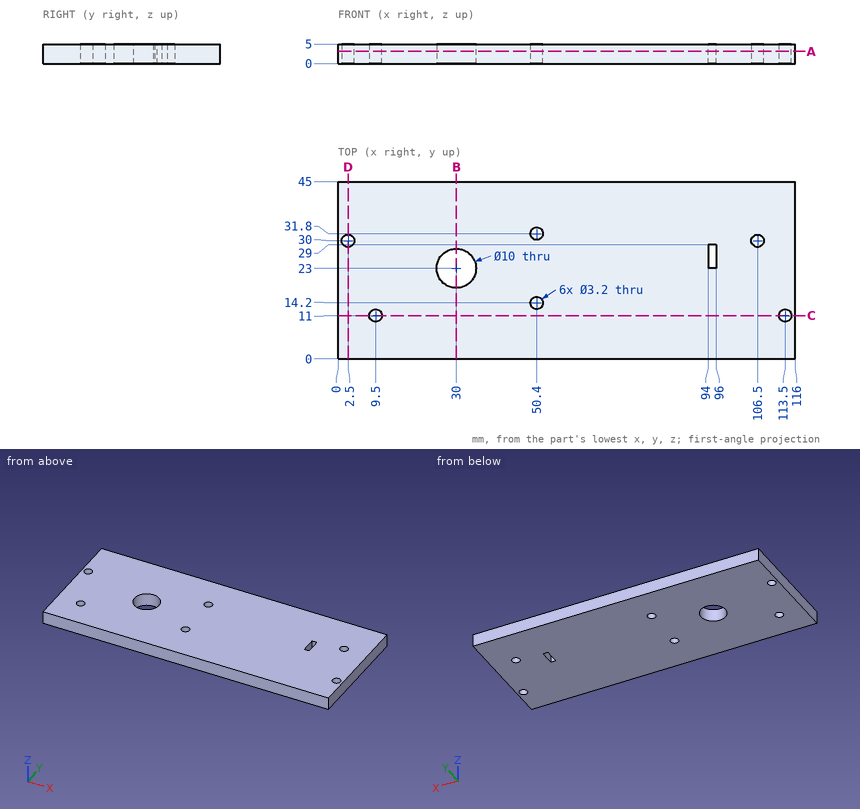
For this review, use the dimensioned drawing (mm, ordinates from the lowest corner) and the shaded views. Give positions to 0.01 mm unless a question says otherwise; leave off trailing zeros. Loops run counter-clockwise (first coordinate to the right, second up) from the corner with the lowest first, then second, coordinate; pieces in that order, holes last. Notation, with made-up numbers: (88.25, 46) -> (98.25, 46) arc R24 ccw to (98.25, 83) -> close; hole circle Ø10 at (7, -21). An arc over 180 degrees is marked (long way). One line per question, with ' | ' between items. Start each with the question number.
(1) We need section B-B (x = 30). State the section outline as (y, z) points, and give its area (3 significant figures).
(2) We need section D-D (x = 2.5). State the section outline as (y, z) points, and give its area (3 significant figures).
(3) We need section A-A (z = 3.15). State how many separate pieces and enclosed holes the cut face has, and give its area (3 significant figures).
(4) We need section C-C (y = 11). State the section outline as (x, z) points.
(5) For line 1 (X direction, y = 30, z = 2.95); line 2 (Y direction, x = 50.4, z = 2.7); line 3 (X direction, y = 11, z = 1.1), list the stretches that pass through material, from the lowest coordinate up.
The answers:
1) outline: (0, 0) -> (18, 0) -> (18, 5) -> (0, 5) -> close; (28, 0) -> (45, 0) -> (45, 5) -> (28, 5) -> close | area: 175 mm^2
2) outline: (0, 0) -> (28.4, 0) -> (28.4, 5) -> (0, 5) -> close; (31.6, 0) -> (45, 0) -> (45, 5) -> (31.6, 5) -> close | area: 209 mm^2
3) separate pieces: 1 | enclosed holes: 8 | area: 5,080 mm^2
4) outline: (0, 0) -> (7.9, 0) -> (7.9, 5) -> (0, 5) -> close; (11.1, 0) -> (111.9, 0) -> (111.9, 5) -> (11.1, 5) -> close; (115.1, 0) -> (116, 0) -> (116, 5) -> (115.1, 5) -> close
5) line 1: x = 0 to 0.9, 4.1 to 104.9, 108.1 to 116 | line 2: y = 0 to 12.6, 15.8 to 30.2, 33.4 to 45 | line 3: x = 0 to 7.9, 11.1 to 111.9, 115.1 to 116
